from build123d import *

# Parameters (mm, degrees)
F0_R     = 2.38125
F0_R_2   = 3.175
F1_DEPTH = 3.175
F3_DEPTH = 3.176
F4_R     = 1.627418
F5_DEPTH = 0.6604


with BuildPart() as f1:
    # F0 (on Front) → F1 (new body)
    with BuildSketch(Plane.XZ):
        with BuildLine():
            ThreePointArc((-30.1244, -15.477998), (-29.078185, -18.003785), (-26.552398, -19.05))
            Line((-26.552398, -19.05), (8.365998, -19.05))
            ThreePointArc((8.365998, -19.05), (10.891785, -18.003785), (11.938, -15.477998))
            Line((11.938, -15.477998), (11.938, 27.999858))
            ThreePointArc((11.938, 27.999858), (10.77674, 31.660388), (7.717692, 33.982074))
            ThreePointArc((7.717692, 33.982074), (5.805787, 35.433129), (5.08, 37.72096))
            Line((5.08, 37.72096), (5.08, 37.9984))
            Line((5.08, 37.9984), (-26.552398, 37.9984))
            ThreePointArc((-26.552398, 37.9984), (-29.078185, 36.952185), (-30.1244, 34.426398))
            Line((-30.1244, 34.426398), (-30.1244, -15.477998))
        make_face()
        with Locations((7.1755, -11.684)):
            Circle(F0_R, mode=Mode.SUBTRACT)
        Circle(F0_R_2, mode=Mode.SUBTRACT)
        with Locations((-23.0124, 33.5534)):
            Circle(F0_R, mode=Mode.SUBTRACT)
        with Locations((-3.9624, 33.5534)):
            Circle(F0_R, mode=Mode.SUBTRACT)
    extrude(amount=F1_DEPTH)

    # F2 (on face) → F3 (cut, through all)
    with BuildSketch(Plane.XZ.offset(3.175)):
        Polygon((0, 6.415805), (-5.55625, 3.207902), (-5.55625, -3.207902), (0, -6.415805), (5.55625, -3.207902), (5.55625, 3.207902), align=None)
    extrude(amount=-F3_DEPTH, mode=Mode.SUBTRACT)

    # F4 (on face) → F5 (cut)
    with BuildSketch(Plane.XZ.offset(3.175)):
        with Locations((-25.760997, 17.07097)):
            Circle(F4_R)
    extrude(amount=-F5_DEPTH, mode=Mode.SUBTRACT)


solid = f1.part
Source: CAD feature listing. Evaluate the final solid. Frame: model axes, mm. A direction names the side the tool comes from. Coordinates: 2 decimals unless noted, no trailing zeros. Write each loop counter-clockwise with the first axis right and the second up, starting at its lowest first coordinate (ties: lowest second). Pieces come first, ordered by that corner, then holes. Notation, with made-up numbers: M 64.25,-0.5 L 107.25,-0.5 A6 ccw 107.25,5.5 Z; hole C 11.25,33 d2. An arc over 180 degrees is marked long. Use a Markdown table: item, result.
1) Mould query, pull axis X, two halves, no side actions, for faces 4 (the flat face through (-11, -2, 37.998)), 5 (the flat face through (-5.556, -2, 0)), 6 (the flat face through (11.938, -2, 6)), 7 (the flat face through (-2.8, -1.6, -4.8)). Classes: pulls with the +X half, pulls with the -X half, needs draft (parallel to the pull), parting line crosses it, or undercut.
Conclusion:
| item | result |
|---|---|
| face 4 | needs draft |
| face 5 | undercut |
| face 6 | pulls with the +X half |
| face 7 | undercut |
2) Section A-A, the plane z = -4.5. Output: boundary loops of the cut face in (x, y) (3 decimals).
Conclusion:
| item | result |
|---|---|
| outline | M -30.124,-3.175 L -3.318,-3.175 L -3.318,0 L -30.124,0 Z; M 3.318,-3.175 L 11.938,-3.175 L 11.938,0 L 3.318,0 Z |
3) Section C-C, the plane x = -4. Output: boundary loops of the cut face in (y, z) (3 decimals), then the cut area to 3 significant figures.
Conclusion:
| item | result |
|---|---|
| outline | M -3.175,-19.05 L 0,-19.05 L 0,-4.106 L -3.175,-4.106 Z; M -3.175,4.106 L 0,4.106 L 0,31.172 L -3.175,31.172 Z; M -3.175,35.934 L 0,35.934 L 0,37.998 L -3.175,37.998 Z |
| area | 140 mm^2 |
4) Section D-D, the plane z = 16.5. Output: boundary loops of the cut face in (x, y) (3 decimals), then the cut area to 3 significant figures.
Conclusion:
| item | result |
|---|---|
| outline | M -30.124,-3.175 L -27.285,-3.175 L -27.285,-2.515 L -24.237,-2.515 L -24.237,-3.175 L 11.938,-3.175 L 11.938,0 L -30.124,0 Z |
| area | 132 mm^2 |
5) Ray query, L1, parallel to Z at x = 5, y = -1.45; L2, parallel to X at y = -2, z = 32; L3, parallel to X at y = -2.15, z = -1. Return the intervals inside material, ascending.
Conclusion:
| item | result |
|---|---|
| L1 | z = -19.05 to -12.65, -10.72 to -3.53, 3.53 to 38 |
| L2 | x = -30.12 to -24.82, -21.21 to -5.77, -2.16 to 10.52 |
| L3 | x = -30.12 to -5.56, 5.56 to 11.94 |
6) Section B-B, the plane y = -0.6. Output: boundary loops of the cut face in (x, z).
Conclusion:
| item | result |
|---|---|
| outline | M -30.12,-15.48 A3.57 ccw -26.55,-19.05 L 8.37,-19.05 A3.57 ccw 11.94,-15.48 L 11.94,28 A6.35 ccw 7.72,33.98 A3.97 cw 5.08,37.72 L 5.08,38 L -26.55,38 A3.57 ccw -30.12,34.43 Z; hole C -23.01,33.55 d4.76; hole C -3.96,33.55 d4.76; hole M -5.56,-3.21 L 0,-6.42 L 5.56,-3.21 L 5.56,3.21 L 0,6.42 L -5.56,3.21 Z; hole C 7.18,-11.68 d4.76 |
7) Reachability of faces 1 (the flat face through (-26, -2.515, 17)), 2 (the flat face through (2.739, -1.61, -4.834)), 3 (the flat face through (-30.124, -2, 10)) from +Z, -Z, +X, -X, +Y, -Y: full face, straight path, thin tool, end or side. Return the list, or none.
Conclusion:
| item | result |
|---|---|
| face 1 | -Y |
| face 2 | +Y, -Y |
| face 3 | +Z, -Z, -X, +Y, -Y |
